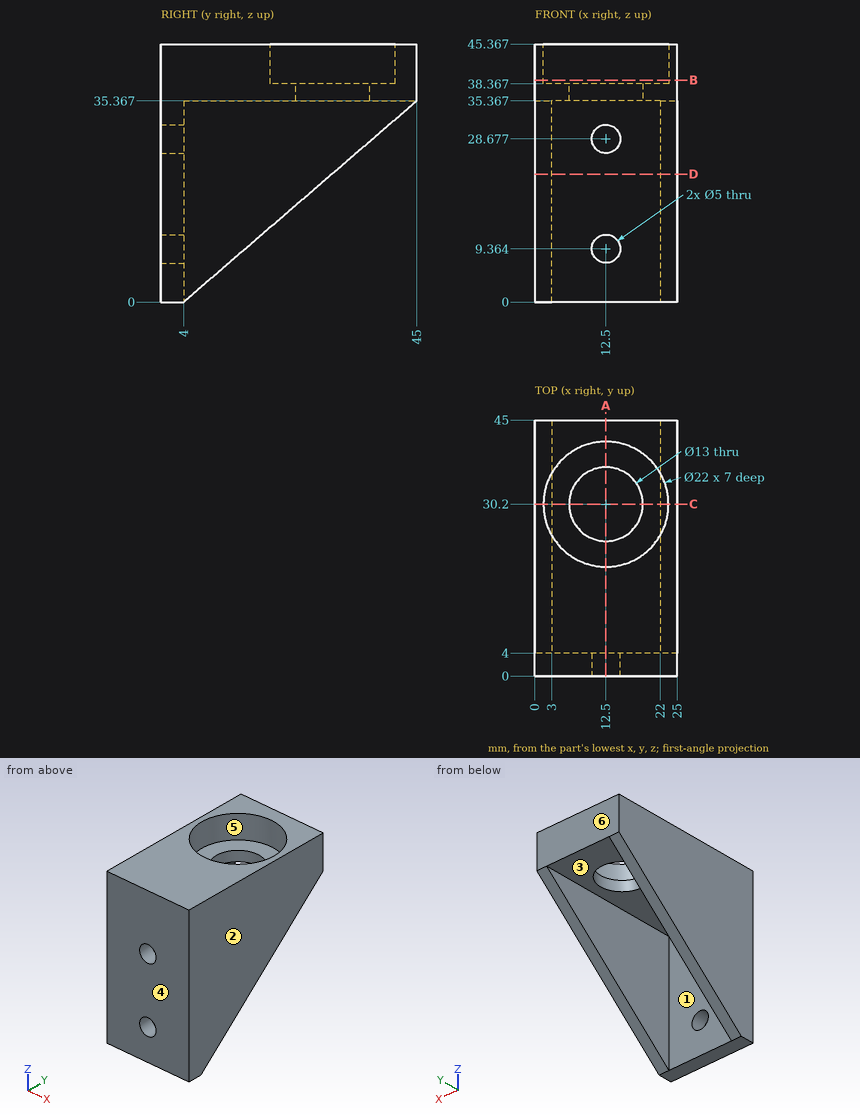
Can you work these out from the drawing? Everything is in mm from the part's minimum corner. A direction names the side the tool comes from. Round coordinates to 2 decimals unless told otherwise and drop trailing zeros. Loops run counter-clockwise (first coordinate to the right, second up) from the corner with the lowest first, then second, coordinate; pieces in that order, holes last. Notation, with made-up numbers: M -26,39 L 12,39 A11 cw 12,59 Z; hole C -16,-34.75 d4. An arc over 180 degrees is marked long. Write item = value, one per line.
1. I want a section at D-D, the plane z = 22.5. Write out the boundary of the cut face in (x, y).
Results below:
outline = M 0,0 L 25,0 L 25,30.08 L 22,30.08 L 22,4 L 3,4 L 3,30.08 L 0,30.08 Z
2. I want a section at C-C, the plane y = 30.2. Write out the boundary of the cut face in (x, z).
Results below:
outline = M 0,22.6 L 3,22.6 L 3,35.37 L 6,35.37 L 6,38.37 L 1.5,38.37 L 1.5,45.37 L 0,45.37 Z; M 19,35.37 L 22,35.37 L 22,22.6 L 25,22.6 L 25,45.37 L 23.5,45.37 L 23.5,38.37 L 19,38.37 Z
3. I want a section at B-B, the plane z = 39. Write out the boundary of the cut face in (x, y).
Results below:
outline = M 0,0 L 25,0 L 25,45 L 0,45 Z; hole C 12.5,30.2 d22
4. Thinking about a two-plate mould opening in Y: for the marked faces 3, 4, 5 and 6, which applies, +Y half, -Y half, draft (parallel to the pull), parting line (faces both ways), or undercut?
Results below:
face_3 = draft
face_4 = -Y half
face_5 = undercut
face_6 = +Y half
5. I want a section at A-A, the plane x = 12.5. Write out the boundary of the cut face in (y, z).
Results below:
outline = M 0,0 L 4,0 L 4,6.86 L 0,6.86 Z; M 0,11.86 L 4,11.86 L 4,26.18 L 0,26.18 Z; M 0,31.18 L 4,31.18 L 4,35.37 L 23.7,35.37 L 23.7,38.37 L 19.2,38.37 L 19.2,45.37 L 0,45.37 Z; M 36.7,35.37 L 45,35.37 L 45,45.37 L 41.2,45.37 L 41.2,38.37 L 36.7,38.37 Z
6. Will these pins go through, and if not, where does the flat tip stop? P1, Ø15, axis at x = 12.5, y = 30.2, coming from the -Z side; P2, Ø11, axis at x = 17, y = 29.5, coming from the +Z side; P3, Ø6.5, axis at x = 12.5, z = 9.36, coming from the +Y side.
Results below:
P1 = 35.37
P2 = 38.37
P3 = 4
7. Which directions (+Z, -Z, +X, -X, +Y, -Y) give clear straight access to the entire face, cutting with the end or side of a thin tool? Please do the marked faces 1 and 2.
Results below:
face_1 = -Z, +Y
face_2 = +Z, -Z, +X, +Y, -Y
8. I need wall thicknesses on probe 1 along Z at (x, y) = (12.5, 2.5); probe 2 along X at (y, z) = (23.5, 34.5); probe 3 along X at (y, z) = (30, 40). Which ranges of each line are inside material? Lowest first, please.
Results below:
probe_1 = 0 to 6.86, 11.86 to 26.18, 31.18 to 45.37
probe_2 = 0 to 3, 22 to 25
probe_3 = 0 to 1.5, 23.5 to 25
